from build123d import *

# Parameters (mm, degrees)
SKETCH1_R                = 8
SKETCH1_R_2              = 4
BOSS_EXTRUDE1_DEPTH      = 9
BOSS_EXTRUDE1_2_DEPTH    = 9
SKETCH2_R                = 4
BOSS_EXTRUDE3_DEPTH      = 9
FILLET1_R                = 1
CUT_EXTRUDE1_DEPTH       = 214.789616212
SKETCH4_W                = 9
SKETCH4_H                = 27
BOSS_EXTRUDE4_DEPTH      = 75
BOSS_EXTRUDE5_START      = 9
SKETCH5_R                = 25
SKETCH5_R_2              = 4
BOSS_EXTRUDE5_DEPTH      = 9
BOSS_EXTRUDE6_DEPTH      = 4.5
BOSS_EXTRUDE6_DEPTH_BACK = 4.5
BOSS_EXTRUDE7_DEPTH      = 4.5
BOSS_EXTRUDE7_DEPTH_BACK = 4.5
BOSS_EXTRUDE7_START      = -25
SKETCH9_W                = 9
SKETCH9_H                = 7
SKETCH9_H_2              = 9
CUT_EXTRUDE2_DEPTH       = 217.612557346
CUT_EXTRUDE3_DEPTH       = 216.299790989
CUT_EXTRUDE3_DEPTH_BACK  = 216.299790989
CAVITY1_START            = -66
CAVITY1_OUTLINE_W        = 9
CAVITY1_OUTLINE_H        = 9
CAVITY1_DEPTH            = 26.25
CAVITY1_START_2          = -35.25
CAVITY1_2_OUTLINE_W      = 9
CAVITY1_2_OUTLINE_H      = 9
CAVITY1_2_DEPTH          = 26.25
CAVITY1_START_3          = -56
CAVITY1_3_OUTLINE_W      = 4.5
CAVITY1_3_OUTLINE_H      = 9
CAVITY1_3_OUTLINE_W_2    = 9
CAVITY1_3_DEPTH          = 9
CAVITY1_START_4          = -28
CAVITY1_4_OUTLINE_W      = 4.5
CAVITY1_4_OUTLINE_H      = 9
CAVITY1_4_OUTLINE_W_2    = 9
CAVITY1_4_DEPTH          = 9


# Read off the part's stored shape, not the designer's step: Cavity1
with BuildPart() as part:
    # Sketch1 → Boss-Extrude1 (new body)
    with BuildSketch(Plane.XY):
        with Locations((-125, 0)):
            Circle(SKETCH1_R)
        with Locations((-125, 0)):
            Circle(SKETCH1_R_2, mode=Mode.SUBTRACT)
    extrude(amount=BOSS_EXTRUDE1_DEPTH)



with BuildPart() as body_2:
    # Sketch1 → Boss-Extrude1 2 (new body)
    with BuildSketch(Plane.XY):
        with Locations((125, 0)):
            Circle(SKETCH1_R)
        with Locations((125, 0)):
            Circle(SKETCH1_R_2, mode=Mode.SUBTRACT)
    extrude(amount=BOSS_EXTRUDE1_2_DEPTH)


with BuildPart() as part_1:
    add(part.part)

    add(body_2.part)  # Boss-Extrude3 merges body 2
    # Sketch2 → Boss-Extrude3 (add)
    with BuildSketch(Plane.XY):
        with BuildLine():
            Line((-175, -75), (125, -75))
            ThreePointArc((125, -75), (130.131670325, -43.377223009), (145.000000492, -14.999999344))
            ThreePointArc((145.000000492, -14.999999344), (143.981414944, 16.269784471), (113.235294528, 22.058823748))
            ThreePointArc((113.235294528, 22.058823748), (25.000000075, 0), (-63.235294395, 22.058823677))
            ThreePointArc((-63.235294395, 22.058823677), (-75.420498385, 24.996463372), (-87.499999896, 21.650635154))
            ThreePointArc((-87.499999896, 21.650635154), (-99.999999954, 18.301270189), (-112.500000024, 21.650635108))
            ThreePointArc((-112.500000024, 21.650635108), (-124.99999995, 25), (-137.49999989, 21.650635158))
            ThreePointArc((-137.49999989, 21.650635158), (-149.999999954, 18.301270189), (-162.50000003, 21.650635112))
            ThreePointArc((-162.50000003, 21.650635112), (-193.705072901, 16.586749162), (-195.000000551, -14.999999265))
            ThreePointArc((-195.000000551, -14.999999265), (-180.13167034, -43.377222962), (-175, -75))
        make_face()
        with Locations((125, 0)):
            Circle(SKETCH2_R, mode=Mode.SUBTRACT)
        with Locations((-175, 0)):
            Circle(SKETCH2_R, mode=Mode.SUBTRACT)
        with Locations((-125, 0)):
            Circle(SKETCH2_R, mode=Mode.SUBTRACT)
        with Locations((-75, 0)):
            Circle(SKETCH2_R, mode=Mode.SUBTRACT)
    extrude(amount=BOSS_EXTRUDE3_DEPTH)

    # Fillet1
    fillet1_edges = [part_1.edges().sort_by_distance(p)[0] for p in [
        (-175, -75, 4.5),
        (125, -75, 4.5),
    ]]
    fillet(fillet1_edges, radius=FILLET1_R)

    # Sketch3 → Cut-Extrude1 (cut, through all)
    with BuildSketch(Plane.XY):
        Polygon((25, 0), (25, -75), (150, -75), (150, 25), (25, 25), align=None)
    extrude(amount=CUT_EXTRUDE1_DEPTH, mode=Mode.SUBTRACT)

    # Sketch4 → Boss-Extrude4 (add)
    with BuildSketch(Plane.XZ.offset(75)):
        with Locations((25, -4.5)):
            Rectangle(SKETCH4_W, SKETCH4_H)
    extrude(amount=-BOSS_EXTRUDE4_DEPTH)

    # Sketch5 → Boss-Extrude5 (add)
    # profile 1 of 4: a face of its own
    with BuildSketch(Plane(origin=(0, 0, -18), x_dir=(-1, 0, 0), z_dir=(0, 0, -1)).offset(BOSS_EXTRUDE5_START)):
        with BuildLine():
            ThreePointArc((-145.000000304, -14.999999594), (-130.131670275, -43.377223158), (-125, -75))
            Line((-125, -75), (-29.5, -75))
            Line((-29.5, -75), (-29.5, 0))
            Line((-29.5, 0), (-100, 0))
            ThreePointArc((-100, 0), (-117.09430609, -23.717082532), (-145.000000304, -14.999999594))
        make_face()
    # profile 2 of 4: a face of its own
    with BuildSketch(Plane(origin=(0, 0, -18), x_dir=(-1, 0, 0), z_dir=(0, 0, -1)).offset(BOSS_EXTRUDE5_START)):
        with Locations((-125, 0)):
            Circle(SKETCH5_R)
        with Locations((-125, 0)):
            Circle(SKETCH5_R_2, mode=Mode.SUBTRACT)
    # profile 3 of 4: a face of its own
    with BuildSketch(Plane(origin=(0, 0, -18), x_dir=(-1, 0, 0), z_dir=(0, 0, -1)).offset(BOSS_EXTRUDE5_START)):
        Polygon((-29.5, 0), (-29.5, -75), (-20.5, -75), (-20.5, 0), (-25, 0), align=None)
    # profile 4 of 4: a face of its own
    with BuildSketch(Plane(origin=(0, 0, -18), x_dir=(-1, 0, 0), z_dir=(0, 0, -1)).offset(BOSS_EXTRUDE5_START)):
        with BuildLine():
            Line((-100, 0), (-29.5, 0))
            Line((-29.5, 0), (-25, 0))
            ThreePointArc((-25, 0), (-70.475429529, 5.598281181), (-113.235293817, 22.058823369))
            ThreePointArc((-113.235293817, 22.058823369), (-103.56267677, 12.86239374), (-100, 0))
        make_face()
    extrude(amount=-BOSS_EXTRUDE5_DEPTH)

    # Sketch7 → Boss-Extrude6 (add, two sides: drawn at the far end of the back side and taken through both)
    with BuildSketch(Plane(origin=(0, -25, 0), x_dir=(1, 0, 0), z_dir=(0, 1, 0)).offset(-BOSS_EXTRUDE6_DEPTH_BACK)):
        with BuildLine():
            Line((56.5, 18), (29.5, 18))
            Line((29.5, 18), (29.5, -9))
            ThreePointArc((29.5, -9), (48.591883092, -1.091883092), (56.5, 18))
        make_face()
        with BuildLine():
            Line((-6.5, 0), (20.5, 0))
            Line((20.5, 0), (20.5, 27))
            ThreePointArc((20.5, 27), (1.408116908, 19.091883092), (-6.5, 0))
        make_face()
    extrude(amount=BOSS_EXTRUDE6_DEPTH + BOSS_EXTRUDE6_DEPTH_BACK)

    # Sketch7<3> → Boss-Extrude7 (add, two sides: drawn at the far end of the back side and taken through both)
    with BuildSketch(Plane(origin=(0, -25, 0), x_dir=(1, 0, 0), z_dir=(0, 1, 0)).offset(BOSS_EXTRUDE7_START - BOSS_EXTRUDE7_DEPTH_BACK)):
        with BuildLine():
            Line((56.5, 18), (29.5, 18))
            Line((29.5, 18), (29.5, -9))
            ThreePointArc((29.5, -9), (48.591883092, -1.091883092), (56.5, 18))
        make_face()
        with BuildLine():
            Line((-6.5, 0), (20.5, 0))
            Line((20.5, 0), (20.5, 27))
            ThreePointArc((20.5, 27), (1.408116908, 19.091883092), (-6.5, 0))
        make_face()
    extrude(amount=BOSS_EXTRUDE7_DEPTH + BOSS_EXTRUDE7_DEPTH_BACK)

    # Sketch9 → Cut-Extrude2 (cut, through all)
    with BuildSketch(Plane.XY.offset(9)):
        with Locations((-160.208548161, -53.5)):
            Rectangle(SKETCH9_W, SKETCH9_H)
        with Locations((-160.208548161, -70.5)):
            Rectangle(SKETCH9_W, SKETCH9_H_2)
        with Locations((-25.351798772, -53.5)):
            Rectangle(SKETCH9_W, SKETCH9_H)
        with Locations((-25.351798772, -70.5)):
            Rectangle(SKETCH9_W, SKETCH9_H_2)
        with Locations((109.504950616, -53.5)):
            Rectangle(SKETCH9_W, SKETCH9_H)
        with Locations((109.504950616, -70.5)):
            Rectangle(SKETCH9_W, SKETCH9_H_2)
    extrude(amount=-CUT_EXTRUDE2_DEPTH, mode=Mode.SUBTRACT)

    # Sketch10 → Cut-Extrude3 (cut, two sides: drawn at the far end of the back side and taken through both)
    with BuildSketch(Plane(origin=(0, 0, 0), x_dir=(1, 0, 0), z_dir=(0, 1, 0)).offset(-CUT_EXTRUDE3_DEPTH_BACK)):
        Polygon((-200, 27), (-200, 0), (29.5, 0), (29.5, -9), (150, -9), (150, 18), (20.5, 18), (20.5, 27), align=None)
    extrude(amount=CUT_EXTRUDE3_DEPTH + CUT_EXTRUDE3_DEPTH_BACK, mode=Mode.SUBTRACT)


with BuildPart() as cut_extrude3_kept_piece:
    # of the separate pieces the step leaves, the one the design keeps (cut_extrude3_pieces_kept)
    add(part_1.part.solids().sort_by_distance((-175.0049016, -74.00990099, 0))[0])

    # Cavity1 outline → Cavity1 (cut)
    with BuildSketch(Plane(origin=(0, 0, 0), x_dir=(1, 0, 0), z_dir=(0, 1, 0)).offset(CAVITY1_START)):
        with Locations((25, -4.5)):
            Rectangle(CAVITY1_OUTLINE_W, CAVITY1_OUTLINE_H)
    extrude(amount=CAVITY1_DEPTH, mode=Mode.SUBTRACT)

    # Cavity1 2 outline → Cavity1 2 (cut)
    with BuildSketch(Plane(origin=(0, 0, 0), x_dir=(1, 0, 0), z_dir=(0, 1, 0)).offset(CAVITY1_START_2)):
        with Locations((25, -4.5)):
            Rectangle(CAVITY1_2_OUTLINE_W, CAVITY1_2_OUTLINE_H)
    extrude(amount=CAVITY1_2_DEPTH, mode=Mode.SUBTRACT)

    # Cavity1 3 outline → Cavity1 3 (cut)
    with BuildSketch(Plane(origin=(0, 0, 0), x_dir=(1, 0, 0), z_dir=(0, 1, 0)).offset(CAVITY1_START_3)):
        with Locations((9.25, -4.5)):
            Rectangle(CAVITY1_3_OUTLINE_W, CAVITY1_3_OUTLINE_H)
        with Locations((-2, -4.5)):
            Rectangle(CAVITY1_3_OUTLINE_W_2, CAVITY1_3_OUTLINE_H)
    extrude(amount=CAVITY1_3_DEPTH, mode=Mode.SUBTRACT)

    # Cavity1 4 outline → Cavity1 4 (cut)
    with BuildSketch(Plane(origin=(0, 0, 0), x_dir=(1, 0, 0), z_dir=(0, 1, 0)).offset(CAVITY1_START_4)):
        with Locations((9.25, -4.5)):
            Rectangle(CAVITY1_4_OUTLINE_W, CAVITY1_4_OUTLINE_H)
        with Locations((-2, -4.5)):
            Rectangle(CAVITY1_4_OUTLINE_W_2, CAVITY1_4_OUTLINE_H)
    extrude(amount=CAVITY1_4_DEPTH, mode=Mode.SUBTRACT)


solid = cut_extrude3_kept_piece.part
Build history of the part. All positions in model axes, mm. A direction names the side the tool comes from. Give positions to 0.01 mm unless a question says otherwise; leave off trailing zeros. Loops run counter-clockwise (first coordinate to the right, second up) from the corner with the lowest first, then second, coordinate; pieces in that order, holes last. Notation, with made-up numbers: (-12.75, -10) -> (35.25, -10) arc R13 ccw to (35.25, 15) -> close; hole circle Ø11 at (45, 4). An arc over 180 degrees is marked (long way). Answer in a Markdown table with one row per item.
Item 1: Slice it at D-D on x = -46. Write the cut outline in (y, z).
Findings below:
| item | result |
|---|---|
| outline | (-75, 0) -> (13.96, 0) -> (13.96, 9) -> (-75, 9) -> close |
Item 2: Slice it at C-C on x = -160. Write the cut outline in (y, z).
Findings below:
| item | result |
|---|---|
| outline | (-66, 0) -> (-57, 0) -> (-57, 9) -> (-66, 9) -> close; (-50, 0) -> (20.39, 0) -> (20.39, 9) -> (-50, 9) -> close |
Item 3: Flat gauge pins, fed straight in: P1, Ø4.5, axis at y = -53.5, z = 4, coming from the -X side; P2, Ø3, axis at y = 8.5, z = 8, coming from the -X side; P3, Ø4.5, axis at y = -24, z = 2.5, coming from the +X side. Where does each tip first touch, or does it go through?
Findings below:
| item | result |
|---|---|
| P1 | stops at x = -177.86 |
| P2 | stops at x = -199 |
| P3 | stops at x = 20.5 |
Item 4: Probe line 1 along X through (y, z) = (-3, 5.25); line 2 along Y through (x, z) = (-57.5, 1.25); line 3 along Y through (x, z) = (-124, 1). List the from-to ranges inside material, lowest first. Write a range as [from, to].
Findings below:
| item | result |
|---|---|
| line 1 | x = [-199.82, -177.65], [-172.35, -127.65], [-122.35, -77.65], [-72.35, 29.5] |
| line 2 | y = [-75, 19.13] |
| line 3 | y = [-75, -3.87], [3.87, 24.98] |
Item 5: Slice it at B-B on z = 4. Give the number of separate pieces and of enclosed holes in the cut face, plus the area to 3 significant figures.
Findings below:
| item | result |
|---|---|
| separate pieces | 1 |
| enclosed holes | 9 |
| area | 18,500 mm² |
Item 6: Slice it at A-A on x = -125. Write the cut outline in (y, z).
Findings below:
| item | result |
|---|---|
| outline | (-75, 0) -> (-4, 0) -> (-4, 9) -> (-75, 9) -> close; (4, 0) -> (25, 0) -> (25, 9) -> (4, 9) -> close |
Item 7: Mould opens along Y. For faces 5 (the flat face through (29.5, -5, 4)), 6 (the cylindrical face through (-180.43, -42.49, 4.44)), 7 (the flat face through (-2, -47, 4)) say: pulls with the +Y half, pulls with the -Y half, needs draft (parallel to the pull), parting line crosses it, or undercut.
Findings below:
| item | result |
|---|---|
| face 5 | needs draft |
| face 6 | pulls with the -Y half |
| face 7 | undercut |
Item 8: Tool access for faces 1 (the flat face through (-29.852, -71, 5)), 2 (the flat face through (20.5, -22, 5)), 3 (the flat face through (-164.709, -54, 5)), 4 (the flat face through (-87, -26, 9)): list every direction of +Z, -Z, +X, -X, +Y, -Y with a clear straight run to the whole face (end or side of a thin tool).
Findings below:
| item | result |
|---|---|
| face 1 | +Z, -Z, -Y |
| face 2 | +Z, -Z, +X |
| face 3 | +Z, -Z |
| face 4 | +Z, +X, -X, +Y, -Y |
